Input: part model. Units: mm. Frame: model coordinates. Round coordinates to 2 decimals unless told otherwise and drop trailing zeros. Loops run counter-clockwise (first coordinate to the right, second up) from the corner with the lowest first, then second, coordinate; pieces in that order, holes last.
1) Section D-D, the plane z = 32. Return loops of the section in (x, y), and give its area (3 significant figures).
2) Section A-A, the plane z = -31.75. Return loops of the section in (x, y), and give its area (3 significant figures).
3) Section B-B, the plane x = 0.5. Return loops of the section in (y, z), and give its area (3 significant figures).
4) Section C-C, the plane y = -2.5. State how many separate pieces and enclosed holes the cut face has, and give its area (3 significant figures).
5) Ray query, line 1 along X through (y, z) = (3.25, -68); line 2 along Z through (x, y) = (-42, -1.5); line 3 along Z through (x, y) = (-39.5, -5). Return the intervals inside material, ascending.
6) First-contact query: pin 1 (4.5 mm diameter, centred on y = 2, z = -54.5, fed in from +X); pin 2 (5 mm diameter, centred on x = -34, y = -3, fed in from -Z); pin 3 (1.3 mm diameter, centred on x = 100.5, y = -2, fed in from -Z). Flat tips, straight axial feed; report the tip coordinate or a pass-through.
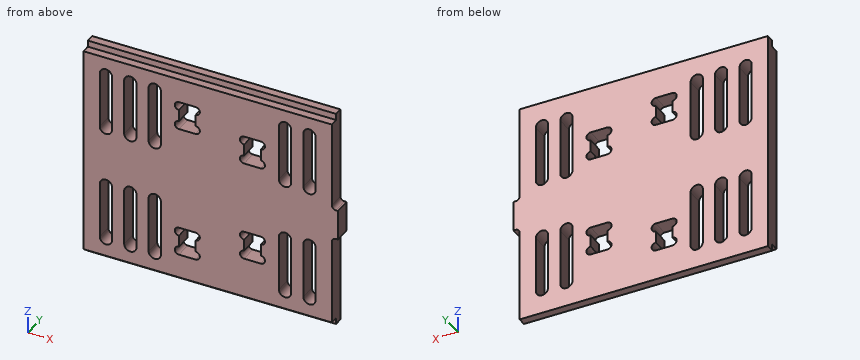
from build123d import *

# Parameters (mm, degrees)
SKETCH1_W           = 175.26
SKETCH1_H           = 12.7
BOSS_EXTRUDE1_DEPTH = 96.8375
SKETCH2_W           = 5.08
SKETCH2_H           = 6.35
CUT_EXTRUDE1_DEPTH  = 213.67191875
CUT_EXTRUDE2_DEPTH  = 132.216646453
CUT_EXTRUDE3_DEPTH  = 132.216646453
SKETCH5_W           = 4.7625
SKETCH5_H           = 23.8125
BOSS_EXTRUDE2_DEPTH = 12.7
FILLET1_R           = 3.175


with BuildPart() as part:
    # Sketch1 → Boss-Extrude1 (new, symmetric)
    with BuildSketch(Plane(origin=(0, 0, 0), x_dir=(0, 0, -1), z_dir=(1, 0, 0))):
        Rectangle(SKETCH1_W, SKETCH1_H)
    extrude(amount=BOSS_EXTRUDE1_DEPTH, both=True)

    # Sketch2 → Cut-Extrude1 (cut, through all)
    with BuildSketch(Plane(origin=(96.8375, 0, 0), x_dir=(0, 0, -1), z_dir=(1, 0, 0))):
        with Locations((-85.09, -3.175)):
            Rectangle(SKETCH2_W, SKETCH2_H)
        with Locations((85.09, -3.175)):
            Rectangle(SKETCH2_W, SKETCH2_H)
    extrude(amount=-CUT_EXTRUDE1_DEPTH, mode=Mode.SUBTRACT)

    # Sketch3 → Cut-Extrude2 (cut, through all)
    with BuildSketch(Plane(origin=(0, 6.35, 0), x_dir=(1, 0, 0), z_dir=(0, 1, 0))):
        with BuildLine():
            Line((28.448, -28.448), (41.402, -28.448))
            ThreePointArc((41.402, -28.448), (44.704, -31.75), (41.402, -35.052))
            Line((41.402, -35.052), (41.402, -44.323))
            ThreePointArc((41.402, -44.323), (44.704, -47.625), (41.402, -50.927))
            Line((41.402, -50.927), (28.448, -50.927))
            ThreePointArc((28.448, -50.927), (25.146, -47.625), (28.448, -44.323))
            Line((28.448, -44.323), (28.448, -35.052))
            ThreePointArc((28.448, -35.052), (25.146, -31.75), (28.448, -28.448))
        make_face()
        with BuildLine():
            Line((-22.352, -41.148), (-9.398, -41.148))
            ThreePointArc((-9.398, -41.148), (-6.096, -44.45), (-9.398, -47.752))
            Line((-9.398, -47.752), (-9.398, -57.023))
            ThreePointArc((-9.398, -57.023), (-6.096, -60.325), (-9.398, -63.627))
            Line((-9.398, -63.627), (-22.352, -63.627))
            ThreePointArc((-22.352, -63.627), (-25.654, -60.325), (-22.352, -57.023))
            Line((-22.352, -57.023), (-22.352, -47.752))
            ThreePointArc((-22.352, -47.752), (-25.654, -44.45), (-22.352, -41.148))
        make_face()
        with BuildLine():
            Line((-9.398, 47.752), (-9.398, 57.023))
            ThreePointArc((-9.398, 57.023), (-6.096, 60.325), (-9.398, 63.627))
            Line((-9.398, 63.627), (-22.352, 63.627))
            ThreePointArc((-22.352, 63.627), (-25.654, 60.325), (-22.352, 57.023))
            Line((-22.352, 57.023), (-22.352, 47.752))
            ThreePointArc((-22.352, 47.752), (-25.654, 44.45), (-22.352, 41.148))
            Line((-22.352, 41.148), (-9.398, 41.148))
            ThreePointArc((-9.398, 41.148), (-6.096, 44.45), (-9.398, 47.752))
        make_face()
        with BuildLine():
            Line((41.402, 35.052), (41.402, 44.323))
            ThreePointArc((41.402, 44.323), (44.704, 47.625), (41.402, 50.927))
            Line((41.402, 50.927), (28.448, 50.927))
            ThreePointArc((28.448, 50.927), (25.146, 47.625), (28.448, 44.323))
            Line((28.448, 44.323), (28.448, 35.052))
            ThreePointArc((28.448, 35.052), (25.146, 31.75), (28.448, 28.448))
            Line((28.448, 28.448), (41.402, 28.448))
            ThreePointArc((41.402, 28.448), (44.704, 31.75), (41.402, 35.052))
        make_face()
    extrude(amount=-CUT_EXTRUDE2_DEPTH, mode=Mode.SUBTRACT)

    # Sketch4 → Cut-Extrude3 (cut, through all)
    with BuildSketch(Plane(origin=(0, 6.35, 0), x_dir=(1, 0, 0), z_dir=(0, 1, 0))):
        with BuildLine():
            Line((55.5625, -68.2625), (55.5625, -23.8125))
            ThreePointArc((55.5625, -23.8125), (60.325, -19.05), (65.0875, -23.8125))
            Line((65.0875, -23.8125), (65.0875, -68.2625))
            ThreePointArc((65.0875, -68.2625), (60.325, -73.025), (55.5625, -68.2625))
        make_face()
        with BuildLine():
            Line((55.5625, 23.8125), (55.5625, 68.2625))
            ThreePointArc((55.5625, 68.2625), (60.325, 73.025), (65.0875, 68.2625))
            Line((65.0875, 68.2625), (65.0875, 23.8125))
            ThreePointArc((65.0875, 23.8125), (60.325, 19.05), (55.5625, 23.8125))
        make_face()
        with BuildLine():
            Line((84.1375, 68.2625), (84.1375, 23.8125))
            ThreePointArc((84.1375, 23.8125), (79.375, 19.05), (74.6125, 23.8125))
            Line((74.6125, 23.8125), (74.6125, 68.2625))
            ThreePointArc((74.6125, 68.2625), (79.375, 73.025), (84.1375, 68.2625))
        make_face()
        with BuildLine():
            Line((84.1375, -23.8125), (84.1375, -68.2625))
            ThreePointArc((84.1375, -68.2625), (79.375, -73.025), (74.6125, -68.2625))
            Line((74.6125, -68.2625), (74.6125, -23.8125))
            ThreePointArc((74.6125, -23.8125), (79.375, -19.05), (84.1375, -23.8125))
        make_face()
        with BuildLine():
            Line((-84.1375, -68.2625), (-84.1375, -23.8125))
            ThreePointArc((-84.1375, -23.8125), (-79.375, -19.05), (-74.6125, -23.8125))
            Line((-74.6125, -23.8125), (-74.6125, -68.2625))
            ThreePointArc((-74.6125, -68.2625), (-79.375, -73.025), (-84.1375, -68.2625))
        make_face()
        with BuildLine():
            Line((-84.1375, 23.8125), (-84.1375, 68.2625))
            ThreePointArc((-84.1375, 68.2625), (-79.375, 73.025), (-74.6125, 68.2625))
            Line((-74.6125, 68.2625), (-74.6125, 23.8125))
            ThreePointArc((-74.6125, 23.8125), (-79.375, 19.05), (-84.1375, 23.8125))
        make_face()
        with BuildLine():
            Line((-65.0875, -68.2625), (-65.0875, -23.8125))
            ThreePointArc((-65.0875, -23.8125), (-60.325, -19.05), (-55.5625, -23.8125))
            Line((-55.5625, -23.8125), (-55.5625, -68.2625))
            ThreePointArc((-55.5625, -68.2625), (-60.325, -73.025), (-65.0875, -68.2625))
        make_face()
        with BuildLine():
            Line((-65.0875, 23.8125), (-65.0875, 68.2625))
            ThreePointArc((-65.0875, 68.2625), (-60.325, 73.025), (-55.5625, 68.2625))
            Line((-55.5625, 68.2625), (-55.5625, 23.8125))
            ThreePointArc((-55.5625, 23.8125), (-60.325, 19.05), (-65.0875, 23.8125))
        make_face()
        with BuildLine():
            Line((-46.0375, -68.2625), (-46.0375, -23.8125))
            ThreePointArc((-46.0375, -23.8125), (-41.275, -19.05), (-36.5125, -23.8125))
            Line((-36.5125, -23.8125), (-36.5125, -68.2625))
            ThreePointArc((-36.5125, -68.2625), (-41.275, -73.025), (-46.0375, -68.2625))
        make_face()
        with BuildLine():
            Line((-46.0375, 23.8125), (-46.0375, 68.2625))
            ThreePointArc((-46.0375, 68.2625), (-41.275, 73.025), (-36.5125, 68.2625))
            Line((-36.5125, 68.2625), (-36.5125, 23.8125))
            ThreePointArc((-36.5125, 23.8125), (-41.275, 19.05), (-46.0375, 23.8125))
        make_face()
    extrude(amount=-CUT_EXTRUDE3_DEPTH, mode=Mode.SUBTRACT)

    # Sketch5 → Boss-Extrude2 (add)
    with BuildSketch(Plane(origin=(0, 6.35, 0), x_dir=(1, 0, 0), z_dir=(0, 1, 0))):
        with Locations((99.21875, 0)):
            Rectangle(SKETCH5_W, SKETCH5_H)
    extrude(amount=-BOSS_EXTRUDE2_DEPTH)

    # Fillet1
    fillet1_edges = [part.edges().sort_by_distance(p)[0] for p in [
        (96.8375, 0, 11.90625),
        (96.8375, 0, -11.90625),
    ]]
    fillet(fillet1_edges, radius=FILLET1_R)


solid = part.part
Final values:
1. outline: (-96.84, -6.35) - (-84.14, -6.35) - (-84.14, 6.35) - (-96.84, 6.35) - close; (-74.61, -6.35) - (-65.09, -6.35) - (-65.09, 6.35) - (-74.61, 6.35) - close; (-55.56, -6.35) - (-46.04, -6.35) - (-46.04, 6.35) - (-55.56, 6.35) - close; (-36.51, -6.35) - (25.16, -6.35) - (25.16, 6.35) - (-36.51, 6.35) - close; (44.69, -6.35) - (55.56, -6.35) - (55.56, 6.35) - (44.69, 6.35) - close; (65.09, -6.35) - (74.61, -6.35) - (74.61, 6.35) - (65.09, 6.35) - close; (84.14, -6.35) - (96.84, -6.35) - (96.84, 6.35) - (84.14, 6.35) - close
1. area: 1,610 mm2
2. outline: (-96.84, -6.35) - (-84.14, -6.35) - (-84.14, 6.35) - (-96.84, 6.35) - close; (-74.61, -6.35) - (-65.09, -6.35) - (-65.09, 6.35) - (-74.61, 6.35) - close; (-55.56, -6.35) - (-46.04, -6.35) - (-46.04, 6.35) - (-55.56, 6.35) - close; (-36.51, -6.35) - (25.15, -6.35) - (25.15, 6.35) - (-36.51, 6.35) - close; (44.7, -6.35) - (55.56, -6.35) - (55.56, 6.35) - (44.7, 6.35) - close; (65.09, -6.35) - (74.61, -6.35) - (74.61, 6.35) - (65.09, 6.35) - close; (84.14, -6.35) - (96.84, -6.35) - (96.84, 6.35) - (84.14, 6.35) - close
2. area: 1,610 mm2
3. outline: (-6.35, -82.55) - (0, -82.55) - (0, -87.63) - (6.35, -87.63) - (6.35, 87.63) - (0, 87.63) - (0, 82.55) - (-6.35, 82.55) - close
3. area: 2,160 mm2
4. separate pieces: 1
4. enclosed holes: 14
4. area: 25,700 mm2
5. line 1: x = -96.84 to -84.14, -74.61 to -65.09, -55.56 to -46.04, -36.51 to 55.56, 65.09 to 74.61, 84.14 to 96.84
5. line 2: z = -82.55 to -72.97, -19.11 to 19.11, 72.97 to 82.55
5. line 3: z = -82.55 to -72.68, -19.39 to 19.39, 72.68 to 82.55
6. pin 1: stops at x = 96.84
6. pin 2: stops at z = -82.55
6. pin 3: stops at z = -11.91
